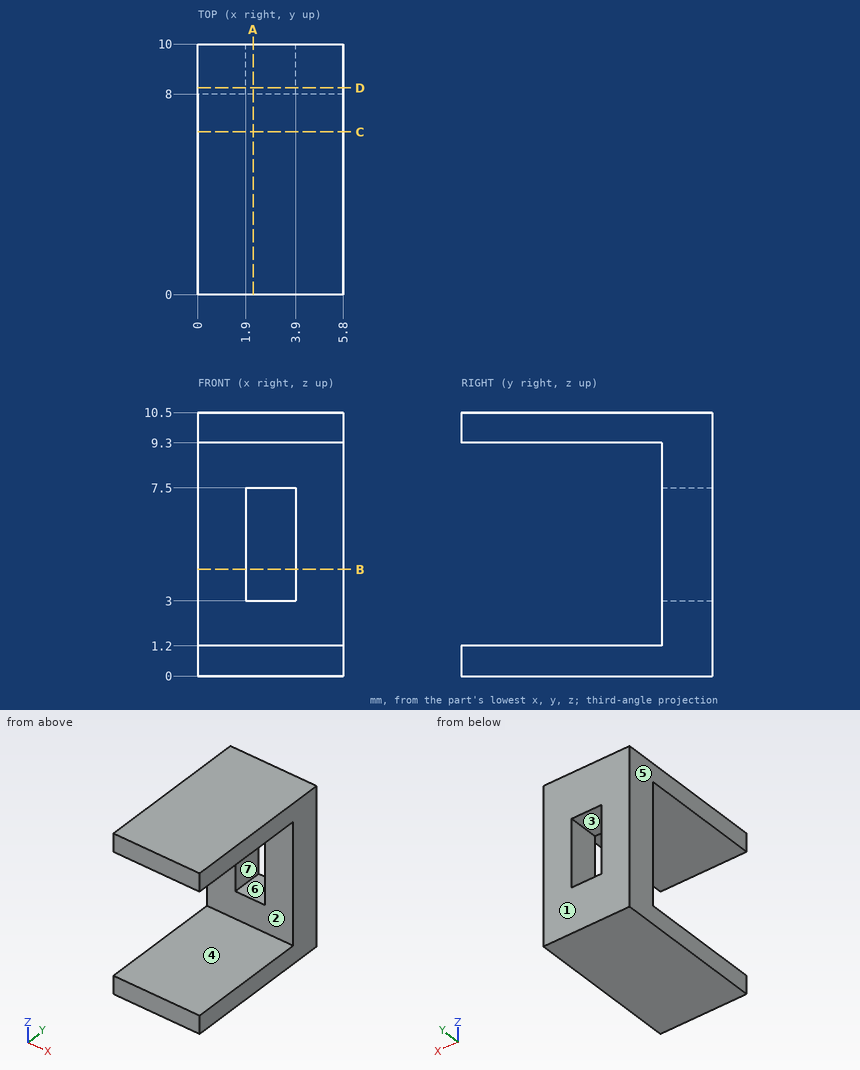
Check sheet for the drawn part. Datum: minimum x, y, z corner. Units: mm. A direction names the side the tool comes from. Give positions to 0.01 mm unless a question says otherwise; leave off trailing zeros. Order: outer loops, then holes, each group sorted by start corner. A loop starts at its lowest first (then second) coordinate and runs counter-clockwise, first axis right, second up. Notation, with made-up numbers: (86, -8) - (97, -8) arc R22 ccw to (97, -2) - close; hole circle Ø1 at (-29.5, 19). An arc over 180 degrees is marked (long way). Answer in a Markdown table with one row per item. Add a question column.
Q1. Material ranges on probe 1 along Z at (x, y) = (4.9, 4.5); probe 2 along Y at (x, z) = (5.5, 5.5), recorded low to high. Write a range as from..to.
Q2. Mould release check, pull along X, two halves, no side actions. Record for the marked faces 4, 5, 6 and 7: pulls with the +X half, pulls with the -X half, needs draft (parallel to the pull), parting line crosses it, or undercut.
Q3. Cross-section at D-D, the plane y = 8.25. Enter the section's corners in (x, z), then the cut area to 3 significant figures.
Q4. Cross-section at C-C, the plane y = 6.5. Enter the section's corners in (x, z).
Q5. Cross-section at B-B, the plane z = 4.25. Enter the section's corners in (x, y).
Q6. Cross-section at A-A, the plane x = 2.2. Enter the section's corners in (y, z).
Q7. Tool access check on the marked faces 1, 2 and 3. Record the directions out of +Z, -Z, +X, -X, +Y, -Y that give a thin tool (end or side, any length) a straight path to the whole face; none if there is none.
Check values:
| question | item | result |
|---|---|---|
| 1 | probe 1 | z = 0..1.2, 9.3..10.5 |
| 1 | probe 2 | y = 8..10 |
| 2 | face 4 | needs draft |
| 2 | face 5 | pulls with the -X half |
| 2 | face 6 | undercut |
| 2 | face 7 | undercut |
| 3 | outline | (0, 0) - (5.8, 0) - (5.8, 10.5) - (0, 10.5) - close; hole (1.9, 3) - (3.9, 3) - (3.9, 7.5) - (1.9, 7.5) - close |
| 3 | area | 51.9 mm^2 |
| 4 | outline | (0, 0) - (5.8, 0) - (5.8, 1.2) - (0, 1.2) - close; (0, 9.3) - (5.8, 9.3) - (5.8, 10.5) - (0, 10.5) - close |
| 5 | outline | (0, 8) - (1.9, 8) - (1.9, 10) - (0, 10) - close; (3.9, 8) - (5.8, 8) - (5.8, 10) - (3.9, 10) - close |
| 6 | outline | (0, 0) - (10, 0) - (10, 3) - (8, 3) - (8, 1.2) - (0, 1.2) - close; (0, 9.3) - (8, 9.3) - (8, 7.5) - (10, 7.5) - (10, 10.5) - (0, 10.5) - close |
| 7 | face 1 | +Z, -Z, +X, -X, +Y |
| 7 | face 2 | +X, -X, -Y |
| 7 | face 3 | +Y, -Y |
